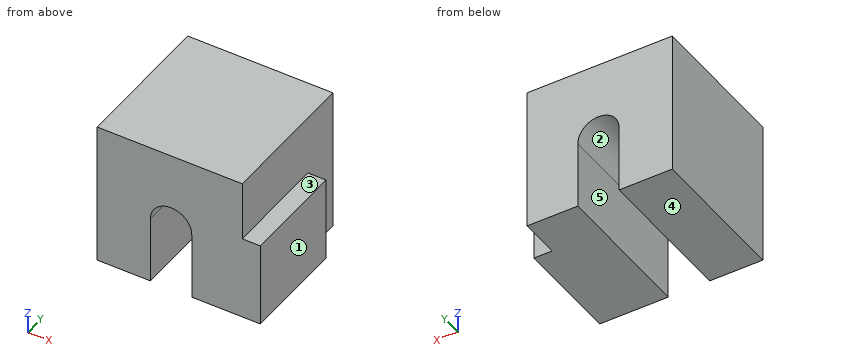
```python
from build123d import *

# Parameters (mm, degrees)
F0_W     = 200
F0_H     = 200
F1_DEPTH = 200
F3_DEPTH = 200
F4_W     = 144.8461644351
F4_H     = 117.3098683357
F5_DEPTH = 25


with BuildPart() as f1:
    # F0 (on Front) → F1 (new body)
    with BuildSketch(Plane.XZ):
        with Locations((56.2296494842, 100)):
            Rectangle(F0_W, F0_H)
    extrude(amount=F1_DEPTH)

    # F2 (on face) → F3 (cut, through all)
    with BuildSketch(Plane.XZ.offset(200)):
        with BuildLine():
            Line((29.5775197446, 93.6536714435), (29.5775197446, 0))
            Line((29.5775197446, 0), (86.5442305803, 0))
            Line((86.5442305803, 0), (86.5442305803, 93.6536714435))
            ThreePointArc((86.5442305803, 93.6536714435), (58.0608751625, 122.1370268613), (29.5775197446, 93.6536714435))
        make_face()
    extrude(amount=-F3_DEPTH, mode=Mode.SUBTRACT)

    # F4 (on face) → F5 (join)
    with BuildSketch(Plane.YZ.offset(156.2296494842)):
        with Locations((-127.5769177824, 58.6549341679)):
            Rectangle(F4_W, F4_H)
    extrude(amount=F5_DEPTH)


solid = f1.part
```
The listing builds one solid part. Answer for the finished solid, in the listing's coordinates (mm). Face numbers are marked on the shaded views. A direction names the side the tool comes from. Give positions to 0.01 mm unless a question says otherwise; leave off trailing zeros. Order: outer loops, then holes, each group sorted by start corner. A loop starts at its lowest first (then second) coordinate and runs counter-clockwise, first axis right, second up. Notation, with made-up numbers: M 80.25,59.5 L 95.25,59.5 A18 cw 95.25,72.5 Z; hole C 87,-28.75 d5. An arc over 180 degrees is marked long. Put each result on its own line as item: value. Start each with the question number.
Item 1: The part is cut by section C-C, the plane z = 176. Determine the outline of the cut face in (x, y).
Item 2: The part is cut by section B-B, the plane y = -14. Determine the outline of the cut face in (x, z).
Item 3: Which of the six approach directions +Z, -Z, +X, -X, +Y, -Y give full straight-line access (tool end or side, diameter ignored) to the marked faces 4 and 5?
Item 4: Find the intervals of material crossed by line 1 along X through (y, z) = (-49.5, 18); line 2 along X through (y, z) = (-101, 33); line 3 along X through (y, z) = (-147, 129), in increasing order.
Item 5: For a pull along X with two mould halves and no side action, classify the marked faces 1, 2 and 3 as +X half, -X half, draft (parallel to the pull), parting line (faces both ways), or undercut.
Item 6: The part is cut by section D-D, the plane x = 48.5. Determine the outline of the cut face in (y, z), and give its area (3 significant figures).
Item 7: The part is cut by section A-A, the plane z = 49. Determine the outline of the cut face in (x, y).
Item 8: Flat-ended cylindrical pins translate along their axes: P1, Ø1.5, axis at y = -35.5, z = 113, coming from the +X side; P2, Ø7.5, axis at x = 171, z = 63, coming from the +Y side. Find the tip coordinate at first contact, or state that the pin passes through.
Answer key:
1. outline: M -43.77,-200 L 156.23,-200 L 156.23,0 L -43.77,0 Z
2. outline: M -43.77,0 L 29.58,0 L 29.58,93.65 A28.48 cw 86.54,93.65 L 86.54,0 L 156.23,0 L 156.23,200 L -43.77,200 Z
3. face 4: -Z, +X, -X, +Y, -Y
3. face 5: -Z, +Y, -Y
4. line 1: x = -43.77 to 29.58, 86.54 to 156.23
4. line 2: x = -43.77 to 29.58, 86.54 to 181.23
4. line 3: x = -43.77 to 156.23
5. face 1: +X half
5. face 2: undercut
5. face 3: draft
6. outline: M -200,120.48 L 0,120.48 L 0,200 L -200,200 Z
6. area: 15,900 mm²
7. outline: M -43.77,-200 L 29.58,-200 L 29.58,0 L -43.77,0 Z; M 86.54,-200 L 181.23,-200 L 181.23,-55.15 L 156.23,-55.15 L 156.23,0 L 86.54,0 Z
8. P1: stops at x = 156.23
8. P2: stops at y = -55.15
